Here's how the part is built. I have some questions about the finished solid (model axes, mm). Face numbers are marked on the shaded views. A direction names the side the tool comes from. Coordinates: 2 decimals unless noted, no trailing zeros. Loops run counter-clockwise (first coordinate to the right, second up) from the corner with the lowest first, then second, coordinate; pieces in that order, holes last. Notation, with made-up numbers: M -17.5,76.5 L 8.5,76.5 A26 ccw 8.5,112.5 Z; hole C 68.5,58 d3. An arc over 180 degrees is marked long. Use one line per item in the form item = value. Start each with the question number.
(1) On a 3-axis mill with a long thin cutter (end or side, diameter ignored), from which of +Z, -Z, +X, -X, +Y, -Y can I reach the whole of each face in a straight line? I mean the marked faces 4, 5 and 6. Say none if no direction works.
(2) Thinking about a two-plate mould opening in Y: for the marked faces 1, 2 and 3, which applies, +Y half, -Y half, draft (parallel to the pull), parting line (faces both ways), or undercut?
(3) Will these pins go through, and if not, where does the flat tip stop? P1, Ø5, axis at x = -51.5, z = 5, coming from the -Y side; P2, Ø3.5, axis at y = 30.5, z = 3.5, coming from the -X side; P3, Ø6, axis at y = 8.5, z = 7.5, coming from the +X side.
(4) Please list where these lines run through material, in increasing order: L1, parallel to Y at x = -37.5, z = 6.5; L2, parallel to X at y = 37.5, z = 1; L3, parallel to Y at x = 51, z = 7.25.
(5) Imagine slicing it at D-D, the plane x = 45.5. Please give me the cut outline in (y, z).
(6) Imagine slicing it at C-C, the plane x = 11.5. Please give me the cut outline in (y, z), and give its area (3 significant figures).
(7) Imagine slicing it at A-A, the plane y = 0. Please give me the cut outline in (x, z), and give its area (3 significant figures).
```python
from build123d import *

# Parameters (mm, degrees)
SKETCH_1_W          = 157
SKETCH_1_H          = 90
EXTRUDE_1_DEPTH     = 13.2
CUT_EXTRUDE_1_DEPTH = 92.441183282
CUT_EXTRUDE_2_DEPTH = 92.441183282
SHELL_1_T           = -1.5
SKETCH_4_R          = 2.5
CUT_EXTRUDE_3_DEPTH = 13.2


with BuildPart() as part:
    # 草图1 → 凸台-拉伸1 (new body)
    with BuildSketch(Plane.XY):
        Rectangle(SKETCH_1_W, SKETCH_1_H)
    extrude(amount=EXTRUDE_1_DEPTH)

    # 草图2 → 切除-拉伸1 (cut, through all)
    with BuildSketch(Plane.XY.offset(13.2)):
        Polygon((-38, 45), (-47.5, 42.25), (-78.5, 42.25), (-78.5, 45), align=None)
        Polygon((78.5, 45), (38, 45), (47.5, 42.25), (78.5, 42.25), align=None)
        Polygon((38, -45), (47.5, -42.25), (78.5, -42.25), (78.5, -45), align=None)
        Polygon((-78.5, -45), (-38, -45), (-47.5, -42.25), (-78.5, -42.25), align=None)
    extrude(amount=-CUT_EXTRUDE_1_DEPTH, mode=Mode.SUBTRACT)

    # 草图3 → 切除-拉伸2 (cut, through all)
    with BuildSketch(Plane.XY.offset(13.2)):
        with BuildLine():
            Line((-68.5, 42.25), (-68.5, 27.25))
            ThreePointArc((-68.5, 27.25), (-78.499, 0), (-68.5, -27.25))
            Line((-68.5, -27.25), (-68.5, -42.25))
            Line((-68.5, -42.25), (-78.5, -42.25))
            Line((-78.5, -42.25), (-78.5, 42.25))
            Line((-78.5, 42.25), (-68.5, 42.25))
        make_face()
        with BuildLine():
            Line((68.5, -42.25), (68.5, -27.25))
            ThreePointArc((68.5, -27.25), (78.499, 0), (68.5, 27.25))
            Line((68.5, 27.25), (68.5, 42.25))
            Line((68.5, 42.25), (78.5, 42.25))
            Line((78.5, 42.25), (78.5, -42.25))
            Line((78.5, -42.25), (68.5, -42.25))
        make_face()
    extrude(amount=-CUT_EXTRUDE_2_DEPTH, mode=Mode.SUBTRACT)

    # 抽壳1
    shell_1_openings = [part.faces().sort_by_distance(p)[0] for p in [
        (0, 0, 0),
    ]]
    offset(amount=SHELL_1_T, openings=shell_1_openings, kind=Kind.INTERSECTION)

    # 草图4 → 切除-拉伸3 (cut)
    with BuildSketch(Plane(origin=(0, 0, 0), x_dir=(-1, 0, 0), z_dir=(0, 0, -1))):
        with Locations((-45.5, 0)):
            Circle(SKETCH_4_R)
        with Locations(Location((45.5, 0, 0), (0, 0, 180))):
            Circle(SKETCH_4_R)
    extrude(amount=-CUT_EXTRUDE_3_DEPTH, mode=Mode.SUBTRACT)


solid = part.part
```
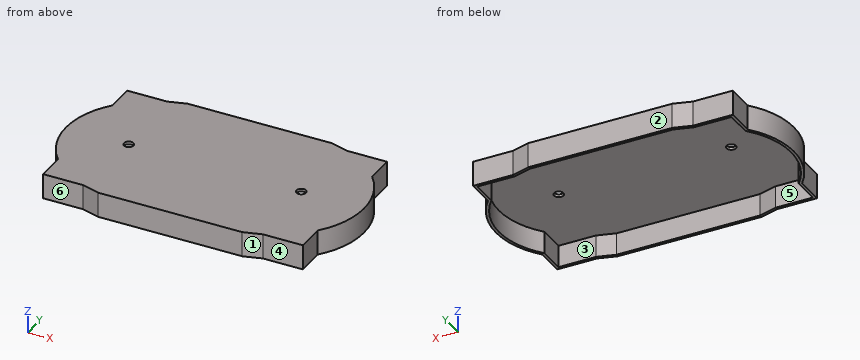
Answer:
q1.face_4 = +Z, -Z, +X, -Y
q1.face_5 = -Z
q1.face_6 = +Z, -Z, -X, -Y
q2.face_1 = -Y half
q2.face_2 = +Y half
q2.face_3 = undercut
q3.P1 = -42.25
q3.P2 = -68.5
q3.P3 = 78.14
q4.L1 = -45 to -43.5, 43.5 to 45
q4.L2 = -68.5 to -67, 67 to 68.5
q4.L3 = -42.25 to -40.75, 40.75 to 42.25
q5.outline = M -42.83,0 L -41.27,0 L -41.27,11.7 L -2.5,11.7 L -2.5,13.2 L -42.83,13.2 Z; M 2.5,11.7 L 41.27,11.7 L 41.27,0 L 42.83,0 L 42.83,13.2 L 2.5,13.2 Z
q6.outline = M -45,0 L -43.5,0 L -43.5,11.7 L 43.5,11.7 L 43.5,0 L 45,0 L 45,13.2 L -45,13.2 Z
q6.area = 170 mm²
q7.outline = M -78.5,0 L -77,0 L -77,11.7 L -48,11.7 L -48,13.2 L -78.5,13.2 Z; M -43,11.7 L 43,11.7 L 43,13.2 L -43,13.2 Z; M 48,11.7 L 77,11.7 L 77,0 L 78.5,0 L 78.5,13.2 L 48,13.2 Z
q7.area = 256 mm²
